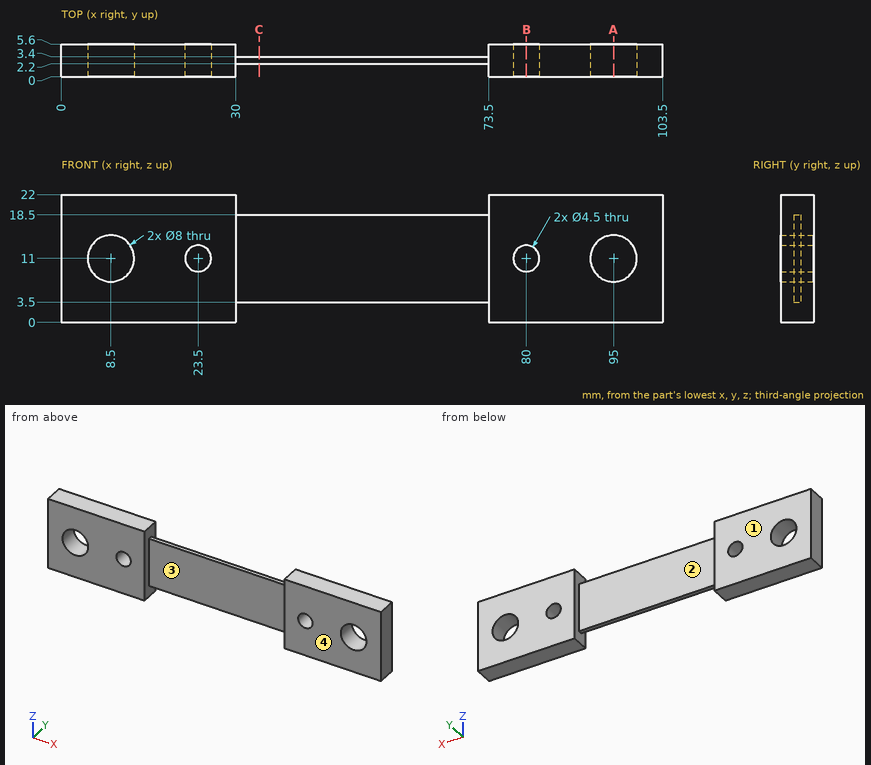
Here's the drawing with two shaded views (mm, measured from the low corner). I have some questions. A direction names the side the tool comes from. Coordinates: 2 decimals unless noted, no trailing zeros. Loops run counter-clockwise (first coordinate to the right, second up) from the corner with the lowest first, then second, coordinate; pieces in that order, holes last. Notation, with made-up numbers: M 20.25,88 L 74.25,88 A31 cw 74.25,127 Z; hole C 68.5,27.5 d3. An arc over 180 degrees is marked long. Answer as CSV lines item,"result". Start each with the question number.
1. Thinking about a two-plate mould opening in X: for the marked faces 3 and 4, which applies, +X half, -X half, draft (parallel to the pull), parting line (faces both ways), or undercut?
2. Suppose I cut it at B-B, the plane x = 80. List the corners of the cut face in (y, z) for me, plus the area to 3 significant figures.
3. Suppose I cut it at A-A, the plane x = 95. List the corners of the cut face in (y, z) for me.
4. For the marked faces 1 and 2, which set-ups out of +Z, -Z, +X, -X, +Y, -Y let a thin tool reach every point of the face, with its end or its side?
5. Suppose I cut it at C-C, the plane x = 34. List the corners of the cut face in (y, z) for me, plus the area to 3 significant figures.
6. If I drill on probe 1 along X at (y, z) = (3.2, 11); probe 2 along X at (y, z) = (1.4, 11); probe 3 along Z at (x, y) = (80, 3.1), over which ranges is the centre line in solid material (lowest first)? Write a range as [from, to].
7. For pin 1 Ø3 at (x, y) = (49.5, 1) entering from +Z; pin 2 Ø1.7 at (y, z) = (2.5, 12.5) entering from -X; pin 3 Ø7.5 at (x, z) = (49.5, 13) entering from -Y; pin 4 Ø7.5 at (x, z) = (52, 11) entering from +Y, each with a flat end and sliding along its axis, tell me the tip position at first contact or that it passes through.
Output:
1,face 3,"undercut"
1,face 4,"draft"
2,outline,"M 0,0 L 5.6,0 L 5.6,8.75 L 0,8.75 Z; M 0,13.25 L 5.6,13.25 L 5.6,22 L 0,22 Z"
2,area,"98.0 mm^2"
3,outline,"M 0,0 L 5.6,0 L 5.6,7 L 0,7 Z; M 0,15 L 5.6,15 L 5.6,22 L 0,22 Z"
4,face 1,"+Z, -Z, +X, -X, +Y"
4,face 2,"+Z, -Z, +Y"
5,outline,"M 2.2,3.5 L 3.4,3.5 L 3.4,18.5 L 2.2,18.5 Z"
5,area,"18.0 mm^2"
6,probe 1,"x = [0, 4.5], [12.5, 21.25], [25.75, 77.75], [82.25, 91], [99, 103.5]"
6,probe 2,"x = [0, 4.5], [12.5, 21.25], [25.75, 30], [73.5, 77.75], [82.25, 91], [99, 103.5]"
6,probe 3,"z = [0, 8.75], [13.25, 22]"
7,pin 1,"stops at z = 18.5"
7,pin 2,"stops at x = 0"
7,pin 3,"stops at y = 2.2"
7,pin 4,"stops at y = 3.4"
